Work out the finished part from the listing and answer in its coordinate system (mm). Face numbers are marked on the shaded views. A direction names the side the tool comes from. Give positions to 0.01 mm unless a question says otherwise; leave off trailing zeros. Loops run counter-clockwise (first coordinate to the right, second up) from the corner with the lowest first, then second, coordinate; pieces in that order, holes last. Notation, with made-up numbers: M 66,34.25 L 96,34.25 A21 ccw 96,59.25 Z; hole C 20.25,-17 d4. An arc over 180 degrees is marked long. Use a Markdown table: item, result.
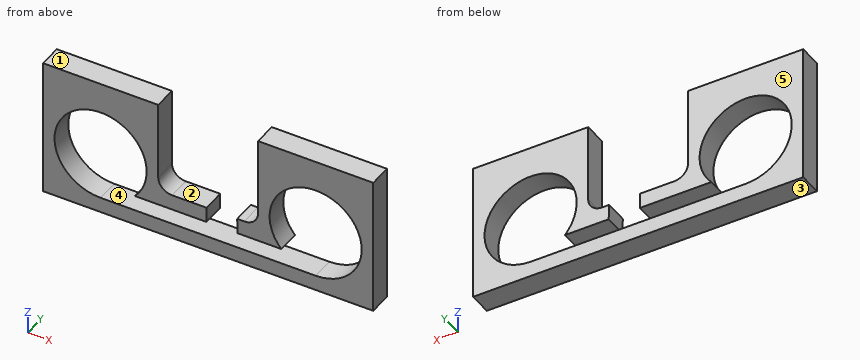
```python
from build123d import *

# Parameters (mm, degrees)
F0_W     = 273.05
F0_H     = 114.3
F1_DEPTH = 19.05
F2_R     = 38.1
F3_DEPTH = 25.4
F5_DEPTH = 25.4
F7_DEPTH = 25.4


with BuildPart() as f1:
    # F0 (on Front) → F1 (new body)
    with BuildSketch(Plane.XZ):
        with Locations((136.525, 57.15)):
            Rectangle(F0_W, F0_H)
    extrude(amount=F1_DEPTH)

    # F2 (on face) → F3 (cut)
    with BuildSketch(Plane.XZ.offset(19.05)):
        with Locations((47.625, 50.8)):
            Circle(F2_R)
        with Locations((225.425, 50.8)):
            Circle(F2_R)
    extrude(amount=-F3_DEPTH, mode=Mode.SUBTRACT)

    # F4 (on face) → F5 (cut)
    with BuildSketch(Plane.XZ.offset(19.05)):
        with BuildLine():
            Line((177.8, 114.3), (95.25, 114.3))
            Line((95.25, 114.3), (95.25, 49.53))
            ThreePointArc((95.25, 49.53), (98.597769, 41.447769), (106.68, 38.1))
            Line((106.68, 38.1), (166.37, 38.1))
            ThreePointArc((166.37, 38.1), (174.452231, 41.447769), (177.8, 49.53))
            Line((177.8, 49.53), (177.8, 114.3))
        make_face()
    extrude(amount=-F5_DEPTH, mode=Mode.SUBTRACT)

    # F6 (on face) → F7 (cut)
    with BuildSketch(Plane.XZ.offset(19.05)):
        Polygon((160.862069, 25.4), (160.547867, 38.1), (135.147867, 38.1), (135.147867, 25.4), (76.023063, 25.4), (47.625, 12.7), (225.425, 12.7), (197.026937, 25.4), align=None)
    extrude(amount=-F7_DEPTH, mode=Mode.SUBTRACT)


solid = f1.part
```
(1) A cutting plane is placed at B-B (x = 232.5). Write down the section's boundary in (y, z).
Entries:
| item | result |
|---|---|
| outline | M -19.05,0 L 0,0 L 0,13.36 L -19.05,13.36 Z; M -19.05,88.24 L 0,88.24 L 0,114.3 L -19.05,114.3 Z |
(2) Which of the six approach directions +Z, -Z, +X, -X, +Y, -Y give full straight-line access (tool end or side, diameter ignored) to the marked faces 1 and 2?
Entries:
| item | result |
|---|---|
| face 1 | +Z, +X, -X, +Y, -Y |
| face 2 | +Z, +Y, -Y |
(3) Given P1, Ø1, axis at x = 97.5, y = -16.5, coming from the +Z side; P2, Ø3, axis at x = 163.5, y = -10, coming from the +Z side, each flat-ended and moving along its own axis, determine where each tip first touches the part or whether it passes through.
Entries:
| item | result |
|---|---|
| P1 | stops at z = 43.45 |
| P2 | stops at z = 38.1 |
(4) A cutting plane is placed at C-C (y = -13.75). Write down the section's boundary in (x, z) (3 decimals), and give its area (3 significant figures).
Entries:
| item | result |
|---|---|
| outline | M 0,0 L 273.05,0 L 273.05,114.3 L 177.8,114.3 L 177.8,49.53 A11.43 cw 166.37,38.1 L 160.548,38.1 L 160.862,25.4 L 197.027,25.4 A38.1 cw long 225.425,12.7 L 47.625,12.7 A38.1 cw long 76.023,25.4 L 135.148,25.4 L 135.148,38.1 L 106.68,38.1 A11.43 cw 95.25,49.53 L 95.25,114.3 L 0,114.3 Z |
| area | 13,800 mm² |
(5) A cutting plane is placed at A-A (z = 107.5). Write down the section's boundary in (x, y).
Entries:
| item | result |
|---|---|
| outline | M 0,-19.05 L 95.25,-19.05 L 95.25,0 L 0,0 Z; M 177.8,-19.05 L 273.05,-19.05 L 273.05,0 L 177.8,0 Z |
(6) A cutting plane is placed at D-D (z = 71). Write down the section's boundary in (x, y), and give its area (3 significant figures).
Entries:
| item | result |
|---|---|
| outline | M 0,-19.05 L 15.32,-19.05 L 15.32,0 L 0,0 Z; M 79.93,-19.05 L 95.25,-19.05 L 95.25,0 L 79.93,0 Z; M 177.8,-19.05 L 193.12,-19.05 L 193.12,0 L 177.8,0 Z; M 257.73,-19.05 L 273.05,-19.05 L 273.05,0 L 257.73,0 Z |
| area | 1,170 mm² |
(7) The mould has two halves that part along Z. Classify the marked faces 3, 4 and 5: released by +Z, released by -Z, zero draft, split by the parting line, or undercut.
Entries:
| item | result |
|---|---|
| face 3 | released by -Z |
| face 4 | undercut |
| face 5 | zero draft |
(8) Consider probe 1 along X at (y, z) = (-3.75, 50.8) (3 decimals); probe 2 along X at (y, z) = (-13, 92); probe 3 along X at (y, z) = (-1.75, 83.5). Determine where each line is inside the solid, lowest interval first. Write a range as [from, to].
Entries:
| item | result |
|---|---|
| probe 1 | x = [0, 9.525], [85.725, 95.25], [177.8, 187.325], [263.525, 273.05] |
| probe 2 | x = [0, 95.25], [177.8, 273.05] |
| probe 3 | x = [0, 28.07], [67.18, 95.25], [177.8, 205.87], [244.98, 273.05] |
